Read the model definition and answer for the solid it produces. Units are mm, in the model's axes. A direction names the side the tool comes from. Coordinates: 2 decimals unless noted, no trailing zeros. Write each loop counter-clockwise with the first axis right and the second up, starting at its lowest first coordinate (ties: lowest second). Pieces come first, ordered by that corner, then holes. Notation, with made-up numbers: (-25, 40) -> (2, 40) arc R23 cw to (2, 50) -> close; hole circle Ø8 at (-2.5, 89). An arc over 180 degrees is marked (long way). One line per item, written item: value. Start each with the question number.
1. For faces 4 (the flat face through (116.5, 104, 55.9)), 5 (the cylindrical face through (72.79, 0.986, 18.562)), 6 (the cylindrical face through (96.2, 3, 60.6)), determine the directions among +Z, -Z, +X, -X, +Y, -Y from which every point of the face is accessible in a straight line to the end or side of a thin tool.
2. Find section D-D, the plane x = 110. Write down the section's boundary in (y, z), and give its area (3 significant figures).
3. Consider line 1 along X through (y, z) = (65.5, 56); line 2 along Z through (x, y) = (137, 73); line 3 along X through (y, z) = (3.1, 56). Determine where each line is inside the solid, lowest interval first.
4. For a pull along Z with two mould halves and no side action, classify faces 1 (the cylindrical face through (151.94, 52.73, 40.52)), 2 (the flat face through (90, 70, 112)), 3 (the flat face through (183, 70, 57)) as pulls with the +Z half, pulls with the -Z half, needs draft (parallel to the pull), parting line crosses it, or undercut.
5. Find section C-C, the plane x = 137.75. Write down the section's boundary in (y, z), and give its area (3 significant figures).
6. Find section B-B, the plane z = 56. Write down the section's boundary in (x, y).
7. Find section A-A, the plane y = 58. Write down the section's boundary in (x, z).
8. Given P1, Ø14.5, axis at x = 127, z = 47.5, coming from the +Y side, flat-ended and moving along its own axis, determine where the tip first touches the part or whether it passes through.
```python
from build123d import *

# Parameters (mm, degrees)
SKETCH1_W           = 183
SKETCH1_H           = 112
BOSS_EXTRUDE1_DEPTH = 4
SKETCH2_W           = 183
SKETCH2_H           = 112
SKETCH2_W_2         = 175
SKETCH2_H_2         = 104
BOSS_EXTRUDE2_DEPTH = 139
SKETCH3_R           = 35.5
CUT_EXTRUDE1_DEPTH  = 4
SKETCH4_R           = 39.25
CUT_EXTRUDE2_DEPTH  = 2
SKETCH5_R           = 21
CUT_EXTRUDE3_DEPTH  = 4
BOSS_EXTRUDE3_START = 100
SKETCH6_R           = 24
SKETCH6_R_2         = 21
BOSS_EXTRUDE3_DEPTH = 100


with BuildPart() as part:
    # Sketch1 → Boss-Extrude1 (new body)
    with BuildSketch(Plane(origin=(0, 0, 0), x_dir=(1, 0, 0), z_dir=(0, 1, 0))):
        with Locations((91.5, -56)):
            Rectangle(SKETCH1_W, SKETCH1_H)
    extrude(amount=BOSS_EXTRUDE1_DEPTH)

    # Sketch2 → Boss-Extrude2 (add)
    with BuildSketch(Plane(origin=(0, 4, 0), x_dir=(1, 0, 0), z_dir=(0, 1, 0))):
        with Locations((91.5, -56)):
            Rectangle(SKETCH2_W, SKETCH2_H)
        with Locations((91.5, -56)):
            Rectangle(SKETCH2_W_2, SKETCH2_H_2, mode=Mode.SUBTRACT)
    extrude(amount=BOSS_EXTRUDE2_DEPTH)

    # Sketch3 → Cut-Extrude1 (cut)
    with BuildSketch(Plane(origin=(0, 0, 0), x_dir=(-1, 0, 0), z_dir=(0, -1, 0))):
        with Locations(Location((-61, -56, 0), (0, 0, 90))):
            Circle(SKETCH3_R)
    extrude(amount=-CUT_EXTRUDE1_DEPTH, mode=Mode.SUBTRACT)

    # Sketch4 → Cut-Extrude2 (cut)
    with BuildSketch(Plane(origin=(0, 0, 0), x_dir=(-1, 0, 0), z_dir=(0, -1, 0))):
        with Locations(Location((-61, -56, 0), (0, 0, 90))):
            Circle(SKETCH4_R)
    extrude(amount=-CUT_EXTRUDE2_DEPTH, mode=Mode.SUBTRACT)

    # Sketch5 → Cut-Extrude3 (cut)
    with BuildSketch(Plane(origin=(0, 4, 0), x_dir=(1, 0, 0), z_dir=(0, 1, 0))):
        with Locations(Location((137.75, -56, 0), (0, 0, 270))):
            Circle(SKETCH5_R)
    extrude(amount=-CUT_EXTRUDE3_DEPTH, mode=Mode.SUBTRACT)

    # Sketch6 → Boss-Extrude3 (add)
    with BuildSketch(Plane(origin=(0, 4, 0), x_dir=(1, 0, 0), z_dir=(0, 1, 0)).offset(BOSS_EXTRUDE3_START)):
        with Locations(Location((137.75, -56, 0), (0, 0, 270))):
            Circle(SKETCH6_R)
        with Locations(Location((137.75, -56, 0), (0, 0, 270))):
            Circle(SKETCH6_R_2, mode=Mode.SUBTRACT)
    extrude(amount=-BOSS_EXTRUDE3_DEPTH)


solid = part.part
```
Answer block:
1. face 4: +Y
1. face 5: -Y
1. face 6: +Y, -Y
2. outline: (0, 0) -> (143, 0) -> (143, 4) -> (4, 4) -> (4, 108) -> (143, 108) -> (143, 112) -> (0, 112) -> close
2. area: 1,560 mm2
3. line 1: x = 0 to 4, 113.75 to 116.75, 158.75 to 161.75, 179 to 183
3. line 2: z = 0 to 4, 32.01 to 35.01, 76.99 to 79.99, 108 to 112
3. line 3: x = 0 to 25.5, 96.5 to 116.75, 158.75 to 183
4. face 1: undercut
4. face 2: pulls with the +Z half
4. face 3: needs draft
5. outline: (0, 0) -> (143, 0) -> (143, 4) -> (4, 4) -> (4, 32) -> (104, 32) -> (104, 35) -> (0, 35) -> close; (0, 77) -> (104, 77) -> (104, 80) -> (4, 80) -> (4, 108) -> (143, 108) -> (143, 112) -> (0, 112) -> close
5. area: 1,990 mm2
6. outline: (0, 0) -> (21.75, 0) -> (21.75, 2) -> (25.5, 2) -> (25.5, 4) -> (4, 4) -> (4, 143) -> (0, 143) -> close; (96.5, 2) -> (100.25, 2) -> (100.25, 0) -> (116.75, 0) -> (116.75, 104) -> (113.75, 104) -> (113.75, 4) -> (96.5, 4) -> close; (158.75, 0) -> (183, 0) -> (183, 143) -> (179, 143) -> (179, 4) -> (161.75, 4) -> (161.75, 104) -> (158.75, 104) -> close
7. outline: (0, 0) -> (183, 0) -> (183, 112) -> (0, 112) -> close; circle Ø48 at (137.75, 56); hole (4, 4) -> (179, 4) -> (179, 108) -> (4, 108) -> close; hole circle Ø42 at (137.75, 56)
8. P1: passes through
